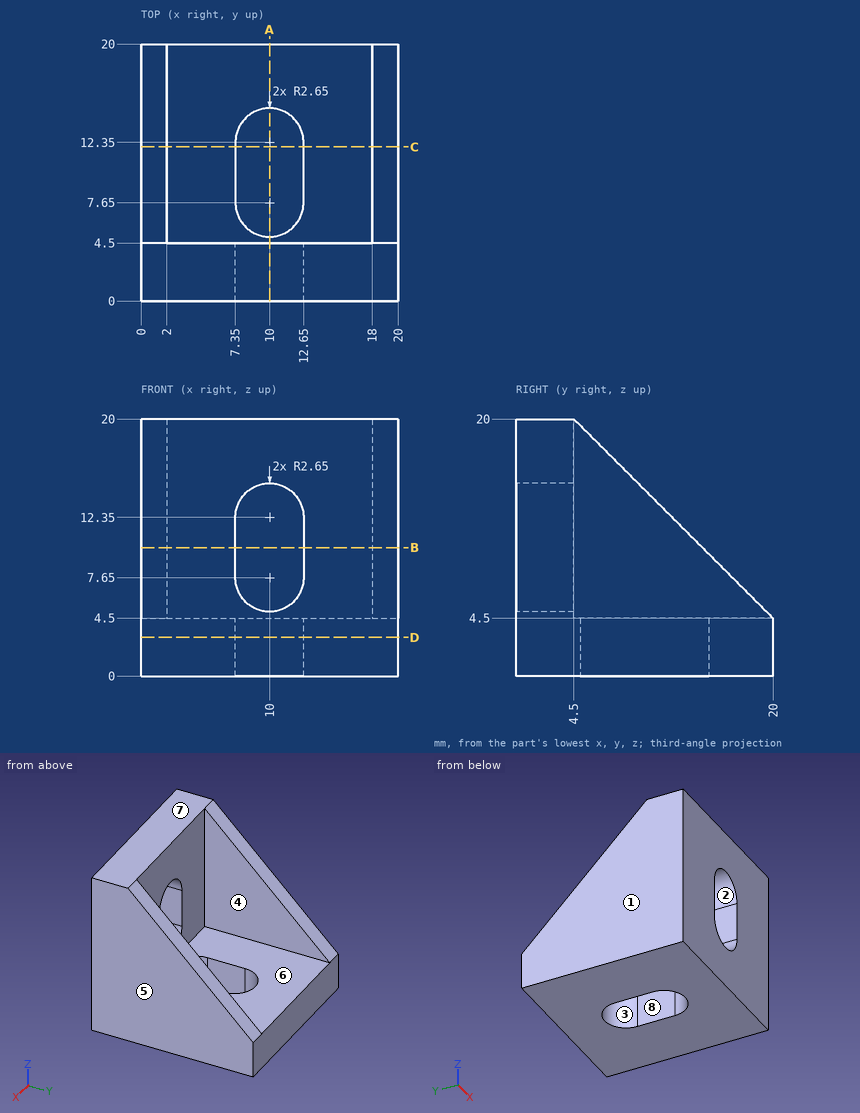
Geometry: see drawing. Coordinates: mm, zero at the bounding-box minimum. A direction names the side the tool comes from. Give positions to 0.01 mm unless a question says otherwise; leave off trailing zeros. Loops run counter-clockwise (first coordinate to the right, second up) from the corner with the lowest first, then second, coordinate; pieces in that order, holes last. Notation, with made-up numbers: (88.5, 29) - (124.5, 29) arc R31 ccw to (124.5, 58) - close; hole circle Ø9 at (-32, 11.25). An arc over 180 degrees is marked (long way). Answer as CSV lines item,"result". Start each with the question number.
1. Section B-B, the plane z = 10. Return loops of the section in (x, y), plus the area to 3 significant figures.
2. Section A-A, the plane x = 10. Return loops of the section in (y, z), plus the area to 4 significant figures.
3. Section C-C, the plane y = 12. Return loops of the section in (x, z), plus the area to 4 significant figures.
4. Draft query along X for the marked faces 5, 6, 7 and 8. Return one class per face: released by +X, released by -X, zero draft, split by the parting line, or undercut.
5. Pin query (flat end, axial travel): P1, Ø4.5, axis at x = 13, z = 10, coming from the +Y side. Return the tip coordinate at first contact, or that it passes through.
6. Reachability of the marked faces 1, 2, 3 and 4 from +Z, -Z, +X, -X, +Y, -Y: full face, straight path, thin tool, end or side. Return the list, or none.
7. Section D-D, the plane z = 3. Return loops of the section in (x, y), plus the area to 3 significant figures.
8. Ray query, L1, parallel to Z at x = 13.5, y = 15.5; L2, parallel to X at y = 6.5, z = 12.5; L3, parallel to X at y = 11.5, z = 2.5. Return the intervals inside material, ascending.
Answers:
1,outline,"(0, 0) - (7.35, 0) - (7.35, 4.5) - (2, 4.5) - (2, 14.5) - (0, 14.5) - close; (12.65, 0) - (20, 0) - (20, 14.5) - (18, 14.5) - (18, 4.5) - (12.65, 4.5) - close"
1,area,"106 mm2"
2,outline,"(0, 0) - (5, 0) - (5, 4.5) - (4.5, 4.5) - (4.5, 5) - (0, 5) - close; (0, 15) - (4.5, 15) - (4.5, 20) - (0, 20) - close; (15, 0) - (20, 0) - (20, 4.5) - (15, 4.5) - close"
2,area,"69.75 mm2"
3,outline,"(0, 0) - (7.35, 0) - (7.35, 4.5) - (2, 4.5) - (2, 12.5) - (0, 12.5) - close; (12.65, 0) - (20, 0) - (20, 12.5) - (18, 12.5) - (18, 4.5) - (12.65, 4.5) - close"
3,area,"98.15 mm2"
4,face 5,"released by +X"
4,face 6,"undercut"
4,face 7,"zero draft"
4,face 8,"undercut"
5,P1,"stops at y = 4.5"
6,face 1,"+Z, -Z, -X, +Y, -Y"
6,face 2,"+Y, -Y"
6,face 3,"+Z, -Z"
6,face 4,"+Z, +Y"
7,outline,"(0, 0) - (20, 0) - (20, 20) - (0, 20) - close; hole (7.35, 7.65) arc R2.65 ccw to (12.65, 7.65) - (12.65, 12.35) arc R2.65 ccw to (7.35, 12.35) - close"
7,area,"353 mm2"
8,L1,"z = 0 to 4.5"
8,L2,"x = 0 to 2, 18 to 20"
8,L3,"x = 0 to 7.35, 12.65 to 20"
